Could you check a few things on this model? Use its own coordinates, in mm. A direction names the side the tool comes from. Coordinates: 2 decimals unless noted, no trailing zeros. Order: outer loops, then holes, each group sorted by start corner. A loop starts at its lowest first (then second) coordinate and runs counter-clockwise, first axis right, second up. Notation, with made-up numbers: (7, 10) - (27, 10) arc R16 cw to (27, 26) - close; hole circle Ø11 at (37, -36). An arc over 180 degrees is marked (long way). One line per item, written item: value. Start each with the question number.
from build123d import *

# Parameters (mm, degrees)
SKETCH1_R           = 6.35
BOSS_EXTRUDE1_DEPTH = 101.6
FILLET1_R           = 1.27
SKETCH2_R           = 3.175
CUT_EXTRUDE1_DEPTH  = 45.72
SKETCH3_R           = 5.08
CUT_EXTRUDE2_DEPTH  = 50.8
FILLET2_R           = 1.27
CUT_EXTRUDE3_DEPTH  = 96.52


with BuildPart() as part:
    # Sketch1 → Boss-Extrude1 (new body)
    with BuildSketch(Plane.XY):
        Circle(SKETCH1_R)
    extrude(amount=BOSS_EXTRUDE1_DEPTH)

    # Fillet1
    fillet1_edges = [part.edges().sort_by_distance(p)[0] for p in [
        (-6.35, 0, 0),
    ]]
    fillet(fillet1_edges, radius=FILLET1_R)

    # Sketch2 → Cut-Extrude1 (cut)
    with BuildSketch(Plane.XY.offset(101.6)):
        Circle(SKETCH2_R)
    extrude(amount=-CUT_EXTRUDE1_DEPTH, mode=Mode.SUBTRACT)

    # Sketch3 → Cut-Extrude2 (cut)
    with BuildSketch(Plane.XY.offset(55.88)):
        Circle(SKETCH3_R)
    extrude(amount=-CUT_EXTRUDE2_DEPTH, mode=Mode.SUBTRACT)

    # Fillet2
    fillet2_edges = [part.edges().sort_by_distance(p)[0] for p in [
        (-6.35, 0, 101.6),
    ]]
    fillet(fillet2_edges, radius=FILLET2_R)

    # Sketch4 → Cut-Extrude3 (cut)
    with BuildSketch(Plane.XY.offset(101.6)):
        with BuildLine():
            Line((-1.27, 6.221703947), (-1.27, 2.909935566))
            Line((-1.27, 2.909935566), (1.27, 2.909935566))
            Line((1.27, 2.909935566), (1.27, 6.221703947))
            ThreePointArc((1.27, 6.221703947), (0, 6.35), (-1.27, 6.221703947))
        make_face()
        with BuildLine():
            Line((2.375061599, 2.107061318), (3.159964765, -0.308622233))
            Line((3.159964765, -0.308622233), (6.309643664, 0.714770478))
            ThreePointArc((6.309643664, 0.714770478), (6.039208878, 1.962257914), (5.524740498, 3.130454029))
            Line((5.524740498, 3.130454029), (2.375061599, 2.107061318))
        make_face()
        with BuildLine():
            Line((2.737868794, -1.607700055), (0.682965628, -3.100674596))
            Line((0.682965628, -3.100674596), (2.629574241, -5.779951497))
            ThreePointArc((2.629574241, -5.779951497), (3.732436352, -5.137257914), (4.684477407, -4.286976956))
            Line((4.684477407, -4.286976956), (2.737868794, -1.607700055))
        make_face()
        with BuildLine():
            Line((-0.682965628, -3.100674596), (-2.737868794, -1.607700055))
            Line((-2.737868794, -1.607700055), (-4.684477407, -4.286976956))
            ThreePointArc((-4.684477407, -4.286976956), (-3.732436352, -5.137257914), (-2.629574241, -5.779951497))
            Line((-2.629574241, -5.779951497), (-0.682965628, -3.100674596))
        make_face()
        with BuildLine():
            Line((-3.159964765, -0.308622233), (-2.375061599, 2.107061318))
            Line((-2.375061599, 2.107061318), (-5.524740498, 3.130454029))
            ThreePointArc((-5.524740498, 3.130454029), (-6.039208878, 1.962257914), (-6.309643664, 0.714770478))
            Line((-6.309643664, 0.714770478), (-3.159964765, -0.308622233))
        make_face()
    extrude(amount=-CUT_EXTRUDE3_DEPTH, mode=Mode.SUBTRACT)


solid = part.part
Q1. I want a section at B-B on z = 47.5. Please give me the cut outline in (x, y), then the cut area to 3 significant figures.
Q2. I'm going to push flat-ended pins straight in: pin 1 (2 mm diameter, centred on y = 3.5, z = 43, fed in from +X); pin 2 (1 mm diameter, centred on y = 4.5, z = 38.5, fed in from -X). Where does each tip first touch, or does it pass through?
Q3. I want a section at A-A on z = 88.5. Please give me the cut outline in (x, y) (3 decimals).
Q4. If I drill on L1, parallel to Z at x = -1.5, y = 4.5; L2, parallel to X at y = 5.75, z = 75.5; L3, parallel to X at y = -3.5, z = 78, over which ranges is the centre line in solid material (lowest first)?
Q5. Which directions (+Z, -Z, +X, -X, +Y, -Y) give clear straight access to the entire face, cutting with the end or side of a thin tool? Please do faces 4 (the flat face through (4.32, 2.74, 64.74)), 5 (the flat face through (-3.914, -3.226, 64.74)), 6 (the flat face through (-5.107, 0.324, 64.74)), 7 (the flat face through (-4, -1, 55.88)).
Q6. We'd pull the mould along Y, two halves only. Please class faces 1 (the flat face through (-1.89, -4.76, 64.74)), 2 (the cylindrical face through (-5.04, -3.86, 50.11)), 3 (the flat face through (-1.27, 5, 65)): +Y half, -Y half, draft (parallel to the pull), parting line (faces both ways), or undercut.
Values follow:
1. outline: (-6.31, 0.71) arc R6.35 ccw to (-4.68, -4.29) - (-3.92, -3.23) arc R5.08 cw to (-5.07, 0.31) - close; (-5.52, 3.13) - (-4.29, 2.73) arc R5.08 cw to (-1.27, 4.92) - (-1.27, 6.22) arc R6.35 ccw to start; (-2.63, -5.78) arc R6.35 ccw to (2.63, -5.78) - (1.86, -4.73) arc R5.08 cw to (-1.86, -4.73) - close; (1.27, 4.92) arc R5.08 cw to (4.29, 2.73) - (5.52, 3.13) arc R6.35 ccw to (1.27, 6.22) - close; (3.92, -3.23) - (4.68, -4.29) arc R6.35 ccw to (6.31, 0.71) - (5.07, 0.31) arc R5.08 cw to start
1. area: 29.3 mm^2
2. pin 1: stops at x = 5.52
2. pin 2: stops at x = -4.93
3. outline: (-6.31, 0.715) arc R6.35 ccw to (-4.684, -4.287) - (-2.738, -1.608) arc R3.175 cw to (-3.16, -0.309) - close; (-5.525, 3.13) - (-2.375, 2.107) arc R3.175 cw to (-1.27, 2.91) - (-1.27, 6.222) arc R6.35 ccw to start; (-2.63, -5.78) arc R6.35 ccw to (2.63, -5.78) - (0.683, -3.101) arc R3.175 cw to (-0.683, -3.101) - close; (1.27, 2.91) arc R3.175 cw to (2.375, 2.107) - (5.525, 3.13) arc R6.35 ccw to (1.27, 6.222) - close; (2.738, -1.608) - (4.684, -4.287) arc R6.35 ccw to (6.31, 0.715) - (3.16, -0.309) arc R3.175 cw to start
4. L1: z = 0 to 5.08, 55.88 to 101.6
4. L2: x = -2.69 to -1.27, 1.27 to 2.69
4. L3: x = -5.3 to -4.11, -0.97 to 0.97, 4.11 to 5.3
5. face 4: +Z, +X
5. face 5: +Z, -Y
5. face 6: +Z
5. face 7: none
6. face 1: undercut
6. face 2: parting line
6. face 3: draft
